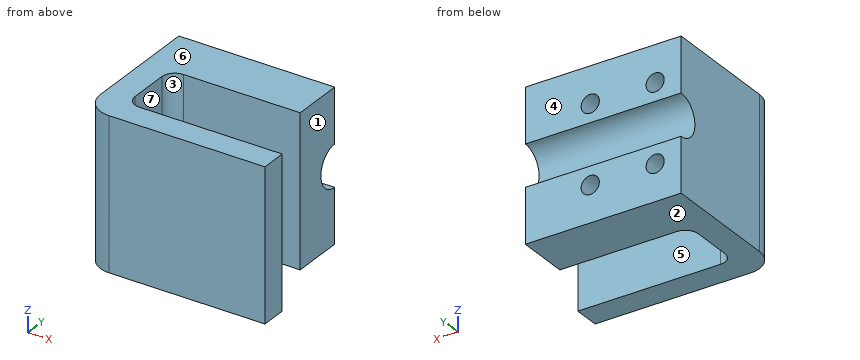
from build123d import *

# Parameters (mm, degrees)
BOSS_EXTRUDE1_DEPTH = 58
SKETCH2_R           = 8
CUT_EXTRUDE1_DEPTH  = 60
SKETCH3_R           = 3.5
CUT_EXTRUDE2_DEPTH  = 18
FILLET1_R           = 5


with BuildPart() as part:
    # Sketch1 → Boss-Extrude1 (new body)
    with BuildSketch(Plane.XY):
        with BuildLine():
            Line((0, 0), (0, 25.5))
            Line((0, 25.5), (50, 25.5))
            Line((50, 25.5), (50, 45.5))
            Line((50, 45.5), (-10, 45.5))
            Line((-10, 45.5), (-10, 0))
            ThreePointArc((-10, 0), (-7.071067812, -7.071067812), (0, -10))
            Line((0, -10), (60, -10))
            Line((60, -10), (60, 0))
            Line((60, 0), (0, 0))
        make_face()
    extrude(amount=BOSS_EXTRUDE1_DEPTH)

    # Sketch2 → Cut-Extrude1 (cut)
    with BuildSketch(Plane.ZY.offset(10)):
        with Locations((29, 45.5)):
            Circle(SKETCH2_R)
    extrude(amount=-CUT_EXTRUDE1_DEPTH, mode=Mode.SUBTRACT)

    # Sketch3 → Cut-Extrude2 (cut)
    with BuildSketch(Plane(origin=(0, 45.5, 0), x_dir=(1, 0, 0), z_dir=(0, 1, 0))):
        with Locations((0, -14)):
            Circle(SKETCH3_R)
        with Locations((0, -44)):
            Circle(SKETCH3_R)
        with Locations((25, -14)):
            Circle(SKETCH3_R)
        with Locations((25, -44)):
            Circle(SKETCH3_R)
    extrude(amount=-CUT_EXTRUDE2_DEPTH, mode=Mode.SUBTRACT)

    # Fillet1
    fillet1_edges = [part.edges().sort_by_distance(p)[0] for p in [
        (0, 25.5, 29),
        (0, 0, 29),
    ]]
    fillet(fillet1_edges, radius=FILLET1_R)


solid = part.part
Design review of the part built by this model. Coordinates are the model's own, in mm. Face numbers are marked on the shaded views. A direction names the side the tool comes from. Coordinates: 2 decimals unless noted, no trailing zeros. Order: outer loops, then holes, each group sorted by start corner. A loop starts at its lowest first (then second) coordinate and runs counter-clockwise, first axis right, second up. Notation, with made-up numbers: (5, 76.5) -> (15, 76.5) arc R21 cw to (15, 90.5) -> close; hole circle Ø7 at (15.25, -15). An arc over 180 degrees is marked (long way). Use one line per item in the form item = value. Start each with the question number.
(1) Add section B-B on y = 41. State the section outline as (x, z) points.
(2) Insertion check: pin 1 (16 mm diameter, centred on y = 38.5, z = 16.5, fed in from +X); pin 2 (6.5 mm diameter, centred on x = 25, z = 44, fed in from +Y); pin 3 (17 mm diameter, centred on y = 14, z = 31.5, fed in from +X). Each pin has a flat end and moves straight along its axis. Give the tip position at first contact, or say it passes through.
(3) The part is to be moulded in two halves that separate along Y. For the marked faces 4, 5, 6 and 7, say which applies: +Y half, -Y half, draft (parallel to the pull), parting line (faces both ways), or undercut.
(4) For the marked faces 1, 2 and 3, list the 3-axis set-ups (+Z, -Z, +X, -X, +Y, -Y) from which the entire face can be reached by the end or side of a thin tool; tool diameter is ignored.
(5) Add section A-A on x = 25. State the section outline as (y, z) points, plus the area to 3 significant figures.
(6) Add section C-C on z = 44. State the section outline as (x, y) points, plus the area to 3 significant figures.
(7) Add section D-D on x = 10.5. State the section outline as (y, z) points.
(8) For probe 1 along X at (y, z) = (35.75, 14); probe 2 along Z at (x, y) = (25, 33); probe 3 along Y at (x, z) = (25, 43), list the stretches that pass through material, from the lowest coordinate up.
Answer block:
q1.outline = (-10, 0) -> (50, 0) -> (50, 22.39) -> (-10, 22.39) -> close; (-10, 35.61) -> (50, 35.61) -> (50, 58) -> (-10, 58) -> close; hole circle Ø7 at (0, 14); hole circle Ø7 at (0, 44); hole circle Ø7 at (25, 14); hole circle Ø7 at (25, 44)
q2.pin_1 = 50
q2.pin_2 = 27.5
q2.pin_3 = 0.42
q3.face_4 = +Y half
q3.face_5 = undercut
q3.face_6 = draft
q3.face_7 = undercut
q4.face_1 = +Z, -Z, +X, +Y
q4.face_2 = -Z, +X, -X, +Y, -Y
q4.face_3 = +Z, -Z, +X
q5.outline = (-10, 0) -> (0, 0) -> (0, 58) -> (-10, 58) -> close; (25.5, 0) -> (45.5, 0) -> (45.5, 10.5) -> (27.5, 10.5) -> (27.5, 17.5) -> (45.5, 17.5) -> (45.5, 21) arc R8 cw to (45.5, 37) -> (45.5, 40.5) -> (27.5, 40.5) -> (27.5, 47.5) -> (45.5, 47.5) -> (45.5, 58) -> (25.5, 58) -> close
q5.area = 1,390 mm²
q6.outline = (-10, 0) arc R10 ccw to (0, -10) -> (60, -10) -> (60, 0) -> (5, 0) arc R5 cw to (0, 5) -> (0, 20.5) arc R5 cw to (5, 25.5) -> (50, 25.5) -> (50, 45.5) -> (28.5, 45.5) -> (28.5, 27.5) -> (21.5, 27.5) -> (21.5, 45.5) -> (3.5, 45.5) -> (3.5, 27.5) -> (-3.5, 27.5) -> (-3.5, 45.5) -> (-10, 45.5) -> close
q6.area = 1,890 mm²
q7.outline = (-10, 0) -> (0, 0) -> (0, 58) -> (-10, 58) -> close; (25.5, 0) -> (45.5, 0) -> (45.5, 21) arc R8 cw to (45.5, 37) -> (45.5, 58) -> (25.5, 58) -> close
q8.probe_1 = -10 to -3.5, 3.5 to 21.5, 28.5 to 50
q8.probe_2 = 0 to 10.5, 17.5 to 40.5, 47.5 to 58
q8.probe_3 = -10 to 0, 25.5 to 27.5
